Design review of the part shown in the three views and the two pictorial views. Dimensions are in mm from the part's minimum x, y and z. A direction names the side the tool comes from. Give positions to 0.01 mm unless a question says otherwise; leave off trailing zeros. Write each loop counter-clockwise with the first axis right and the second up, starting at its lowest first coordinate (ties: lowest second). Pieces come first, ordered by that corner, then holes. Notation, with made-up numbers: M -32.5,9.5 L 3.5,9.5 A19 ccw 3.5,41.5 Z; hole C 25,-1.5 d10. An arc over 180 degrees is marked long. Use one line per item in the form item = value. Start each with the question number.
Q1. Consider section C-C on z = 16.5. Write out the cut boundary in (x, y), and give its area (3 significant figures).
Q2. For probe 1 along X at (y, z) = (12.5, 34.5); probe 2 along X at (y, z) = (9.5, 20); probe 3 along Y at (x, z) = (10, 21), list the stretches that pass through material, from the lowest coordinate up. Write a range as [from, to].
Q3. Clearance check with flat-ended pins moving along their axes: pin 1 Ø4.5 at (y, z) = (8.5, 5.5) entering from -X; pin 2 Ø2 at (x, y) = (13, 6) entering from +Z; pin 3 Ø5 at (x, y) = (7, 11) entering from -Z. State where each tip first meets the part, or that it passes through.
Q4. Consider section D-D on z = 34.5. Write out the cut boundary in (x, y).
Q5. Tool access review of the marked faces 1, 2, 3, 4 and 5: name each direction out of +Z, -Z, +X, -X, +Y, -Y from which nothing blocks a thin tool from reaching the whole face with its end or side.
Q6. Consider section A-A on x = 10. Write out the cut boundary in (y, z), and give its area (3 significant figures).
Q7. Consider section B-B on x = 33. Write out the cut boundary in (y, z).
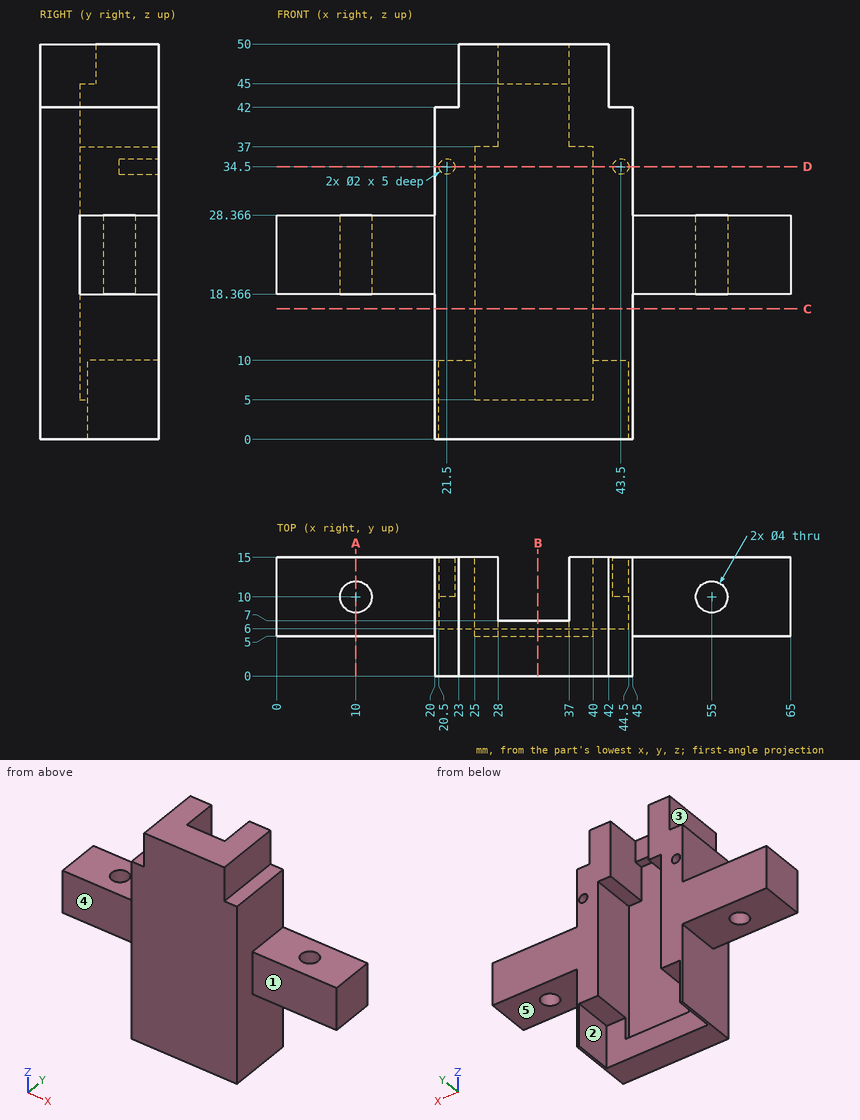
Working result:
q1.outline = M 20,0 L 45,0 L 45,15 L 40,15 L 40,5 L 25,5 L 25,15 L 20,15 Z
q1.area = 225 mm²
q2.probe_1 = [20, 20.5], [22.5, 25], [40, 42.5], [44.5, 45]
q2.probe_2 = [0, 8.06], [11.94, 25], [40, 53.06], [56.94, 65]
q2.probe_3 = [5, 8], [12, 15]
q3.pin_1 = 20
q3.pin_2 = 28.37
q3.pin_3 = 18.37
q4.outline = M 20,0 L 45,0 L 45,15 L 44.5,15 L 44.5,10 L 42.5,10 L 42.5,15 L 40,15 L 40,5 L 25,5 L 25,15 L 22.5,15 L 22.5,10 L 20.5,10 L 20.5,15 L 20,15 Z
q5.face_1 = +Z, -Z, +X, -Y
q5.face_2 = -Z, +Y
q5.face_3 = +Z, -X, +Y, -Y
q5.face_4 = +Z, -Z, -X, -Y
q5.face_5 = -Z, +X, +Y, -Y
q6.outline = M 5,18.37 L 8,18.37 L 8,28.37 L 5,28.37 Z; M 12,18.37 L 15,18.37 L 15,28.37 L 12,28.37 Z
q6.area = 60.0 mm²
q7.outline = M 0,0 L 6,0 L 6,5 L 5,5 L 5,45 L 7,45 L 7,50 L 0,50 Z
